Build history of the part. All positions in model axes, mm. A direction names the side the tool comes from. Coordinates: 2 decimals unless noted, no trailing zeros. Loops run counter-clockwise (first coordinate to the right, second up) from the corner with the lowest first, then second, coordinate; pieces in that order, holes last.
Item 1: Cut at C-C (x = 24). List the corners of the cut face in (y, z).
Item 2: Cut at A-A (z = 0). List the corners of the cut face in (x, y).
Item 3: Mould opens along Z. For faces 1 (the face through (-16.513, -3.131, 74.363)), 2 (the face through (50.936, -3.131, -25.945)), 3 (the face through (-1, 0, -1)) say: released by +Z, released by -Z, zero draft, split by the parting line, or undercut.
Item 4: Cut at D-D (z = 57.15). List the corners of the cut face in (x, y), and give its area (3 significant figures).
Item 5: Flat gauge pins, fed straight in: pin 1 (1 mm diameter, centred on x = -39.5, y = -5.5, fed in from +Z); pin 2 (2 mm diameter, centred on y = -1, z = -2.5, fed in from +X); pin 3 (3 mm diameter, centred on y = -3.5, z = -31, fed in from -X). Where does each tip first touch, or does it go through?
Item 6: Cut at B-B (y = -2.25). List the corners of the cut face in (x, z) (3 decimals), and give its area (3 significant figures).
Item 7: Drill centre lines: line 1 along Z through (x, y) = (18, -2.5); line 2 along Z through (x, y) = (21, -0.75); line 3 along X through (y, z) = (-1, 33). Where is each one in solid material? Low to high.
Item 8: 3-axis set-ups, long thin cutter, end or side, ignore diameter. For faces 4 (the face through (-1, -6.35, -1)), 5 (the face through (30.456, -3.131, -51.87)): which of +Z, -Z, +X, -X, +Y, -Y reach the whole face in a straight line?
from build123d import *

# Parameters (mm, degrees)
SKETCH2_R           = 76.1746
BOSS_EXTRUDE1_DEPTH = 6.35


with BuildPart() as part:
    # Sketch2 → Boss-Extrude1 (new body)
    with BuildSketch(Plane(origin=(0, 0, 0), x_dir=(1, 0, 0), z_dir=(0, 1, 0))):
        Circle(SKETCH2_R)
        with BuildLine():
            ThreePointArc((52.091428011, 30.074999984), (30.074999985, 52.091428011), (0, 60.149999969))
            ThreePointArc((0, 60.149999969), (-2.999999969, 57.15), (0, 54.150000031))
            ThreePointArc((0, 54.150000031), (27.075000016, 46.895275642), (46.895275642, 27.075000015))
            ThreePointArc((46.895275642, 27.075000015), (50.993351811, 25.976923815), (52.091428011, 30.074999984))
        make_face(mode=Mode.SUBTRACT)
        with BuildLine():
            ThreePointArc((0, -54.150000031), (27.075000016, -46.895275642), (46.895275642, -27.075000015))
            ThreePointArc((46.895275642, -27.075000015), (50.993351811, -25.976923815), (52.091428011, -30.074999985))
            ThreePointArc((52.091428011, -30.074999985), (30.074999984, -52.091428011), (0, -60.149999969))
            ThreePointArc((0, -60.149999969), (-2.999999969, -57.15), (0, -54.150000031))
        make_face(mode=Mode.SUBTRACT)
        with BuildLine():
            ThreePointArc((-46.895275642, 27.075000015), (-54.150000031, 0), (-46.895275642, -27.075000016))
            ThreePointArc((-46.895275642, -27.075000016), (-47.993351842, -31.173076185), (-52.091428011, -30.074999985))
            ThreePointArc((-52.091428011, -30.074999985), (-60.149999969, 0), (-52.091428011, 30.074999984))
            ThreePointArc((-52.091428011, 30.074999984), (-47.993351842, 31.173076185), (-46.895275642, 27.075000015))
        make_face(mode=Mode.SUBTRACT)
    extrude(amount=-BOSS_EXTRUDE1_DEPTH)


solid = part.part
Filled sheet:
1. outline: (-6.35, -72.3) - (0, -72.3) - (0, -55.15) - (-6.35, -55.15) - close; (-6.35, -48.54) - (0, -48.54) - (0, 48.54) - (-6.35, 48.54) - close; (-6.35, 55.15) - (0, 55.15) - (0, 72.3) - (-6.35, 72.3) - close
2. outline: (-76.17, -6.35) - (-60.15, -6.35) - (-60.15, 0) - (-76.17, 0) - close; (-54.15, -6.35) - (76.17, -6.35) - (76.17, 0) - (-54.15, 0) - close
3. face 1: split by the parting line
3. face 2: undercut
3. face 3: zero draft
4. outline: (-50.36, -6.35) - (-3, -6.35) - (-3, 0) - (-50.36, 0) - close; (18.76, -6.35) - (50.36, -6.35) - (50.36, 0) - (18.76, 0) - close
4. area: 501 mm2
5. pin 1: stops at z = 65.43
5. pin 2: stops at x = 76.16
5. pin 3: stops at x = -70.23
6. outline: circle Ø152.349 at (0, 0); hole (-52.091, -30.075) arc R3 ccw to (-46.895, -27.075) arc R54.15 cw to (-46.895, 27.075) arc R3 ccw to (-52.091, 30.075) arc R60.15 ccw to start; hole (0, -60.15) arc R60.15 ccw to (52.091, -30.075) arc R3 ccw to (46.895, -27.075) arc R54.15 cw to (0, -54.15) arc R3 ccw to start; hole (0, 54.15) arc R54.15 cw to (46.895, 27.075) arc R3 ccw to (52.091, 30.075) arc R60.15 ccw to (0, 60.15) arc R3 ccw to start
6. area: 17,100 mm2
7. line 1: z = -74.02 to -57.39, -51.07 to 51.07, 57.39 to 74.02
7. line 2: z = -73.22 to -56.37, -49.91 to 49.91, 56.37 to 73.22
7. line 3: x = -68.66 to 42.93, 50.29 to 68.66
8. face 4: +Z, -Z, +X, -X, -Y
8. face 5: +Y, -Y
